Autodesk Inventor part; units mm, degrees
ref_plane "YZ Plane" through (0, 0, 0) normal (1, 0, 0) x (0, 1, 0)
ref_plane "XZ Plane" through (0, 0, 0) normal (0, 1, 0) x (-1, 0, 0)
ref_plane "XY Plane" through (0, 0, 0) normal (0, 0, 1) x (1, 0, 0)
sketch "草圖1" plane through (0, 0, 0) normal (0, 1, 0) x (-1, 0, 0)
  line L0 (21.4547, 24.4389) -> (-48.5453, 24.4389)
  line L1 (0.9998, 25.0567) -> (0.9998, 26.3567)
  line L2 (3.4998, 26.3567) -> (3.4998, 25.0567)
  line L3 (0.9998, 26.3567) -> (3.4998, 26.3567)
  line L4 (3.4998, 25.0567) -> (0.9998, 25.0567)
  line L5 (4.9998, 25.0567) -> (4.9998, 26.3567)
  line L6 (-18.5453, 30.4195) -> (12.788, 30.4195)
  line L7 (7.4998, 26.3567) -> (7.4998, 25.0567)
  line L8 (7.4998, 25.0567) -> (4.9998, 25.0567)
  line L9 (4.9998, 26.3567) -> (7.4998, 26.3567)
  line L10 (8.9998, 25.0567) -> (8.9998, 26.3567)
  line L11 (8.9998, 26.3567) -> (11.4998, 26.3567)
  line L12 (-48.5453, 23.4389) -> (-48.5453, 33.4389)
  line L13 (-38.5108, 33.4389) -> (-38.5108, 32.4389)
  line L14 (-38.5108, 32.4389) -> (-28.5108, 32.4389)
  line L15 (-28.5108, 32.4389) -> (-28.5108, 31.4389)
  line L16 (-18.5453, 31.4389) -> (-18.5453, 30.4195)
  line L17 (-28.5108, 31.4389) -> (-18.5453, 31.4389)
  line L18 (11.4998, 25.0567) -> (8.9998, 25.0567)
  line L19 (-44.5002, 26.3567) -> (-44.5002, 25.0567)
  line L20 (-44.5002, 25.0567) -> (-47.0002, 25.0567)
  line L21 (11.4998, 26.3567) -> (11.4998, 25.0567)
  line L22 (-40.5002, 26.3567) -> (-40.5002, 25.0567)
  line L23 (-40.5002, 25.0567) -> (-43.0002, 25.0567)
  line L24 (-47.0002, 25.0567) -> (-47.0002, 26.3567)
  line L25 (-47.0002, 26.3567) -> (-44.5002, 26.3567)
  line L26 (-43.0002, 26.3567) -> (-40.5002, 26.3567)
  line L27 (-36.5002, 26.3567) -> (-36.5002, 25.0567)
  line L28 (-39.0002, 26.3567) -> (-36.5002, 26.3567)
  line L29 (-39.0002, 25.0567) -> (-39.0002, 26.3567)
  line L30 (-36.5002, 25.0567) -> (-39.0002, 25.0567)
  line L31 (-43.0002, 25.0567) -> (-43.0002, 26.3567)
  line L32 (-32.5002, 26.3567) -> (-32.5002, 25.0567)
  line L33 (-32.5002, 25.0567) -> (-35.0002, 25.0567)
  line L34 (-35.0002, 26.3567) -> (-32.5002, 26.3567)
  line L35 (-35.0002, 25.0567) -> (-35.0002, 26.3567)
  line L36 (-28.5002, 26.3567) -> (-28.5002, 25.0567)
  line L37 (-28.5002, 25.0567) -> (-31.0002, 25.0567)
  line L38 (-31.0002, 26.3567) -> (-28.5002, 26.3567)
  line L39 (-31.0002, 25.0567) -> (-31.0002, 26.3567)
  line L40 (-24.5002, 26.3567) -> (-24.5002, 25.0567)
  line L41 (-24.5002, 25.0567) -> (-27.0002, 25.0567)
  line L42 (-27.0002, 25.0567) -> (-27.0002, 26.3567)
  line L43 (-27.0002, 26.3567) -> (-24.5002, 26.3567)
  line L44 (-20.5002, 26.3567) -> (-20.5002, 25.0567)
  line L45 (-20.5002, 25.0567) -> (-23.0002, 25.0567)
  line L46 (-23.0002, 26.3567) -> (-20.5002, 26.3567)
  line L47 (-23.0002, 25.0567) -> (-23.0002, 26.3567)
  line L48 (-16.5002, 26.3567) -> (-16.5002, 25.0567)
  line L49 (-19.0002, 26.3567) -> (-16.5002, 26.3567)
  line L50 (-19.0002, 25.0567) -> (-19.0002, 26.3567)
  line L51 (-16.5002, 25.0567) -> (-19.0002, 25.0567)
  line L52 (-12.5002, 26.3567) -> (-12.5002, 25.0567)
  line L53 (-15.0002, 26.3567) -> (-12.5002, 26.3567)
  line L54 (-15.0002, 25.0567) -> (-15.0002, 26.3567)
  line L55 (-12.5002, 25.0567) -> (-15.0002, 25.0567)
  line L56 (-8.5002, 26.3567) -> (-8.5002, 25.0567)
  line L57 (-8.5002, 25.0567) -> (-11.0002, 25.0567)
  line L58 (-11.0002, 25.0567) -> (-11.0002, 26.3567)
  line L59 (-11.0002, 26.3567) -> (-8.5002, 26.3567)
  line L60 (-4.5002, 25.0567) -> (-7.0002, 25.0567)
  line L61 (-7.0002, 26.3567) -> (-4.5002, 26.3567)
  line L62 (-7.0002, 25.0567) -> (-7.0002, 26.3567)
  line L63 (-4.5002, 26.3567) -> (-4.5002, 25.0567)
  line L64 (-3.0002, 25.0567) -> (-3.0002, 26.3567)
  line L65 (-0.5002, 25.0567) -> (-3.0002, 25.0567)
  line L66 (-3.0002, 26.3567) -> (-0.5002, 26.3567)
  line L67 (-0.5002, 26.3567) -> (-0.5002, 25.0567)
  line L68 (-48.5453, 33.4389) -> (-38.5108, 33.4389)
  line L69 (21.4547, 24.4389) -> (12.788, 30.4195)
  line L70 (12.2792, 28.0771) -> (12.2792, 25.0771)
  line L71 (14.7792, 28.0771) -> (12.2792, 28.0771)
  line L72 (12.2792, 25.0771) -> (14.7792, 25.0771)
  line L73 (14.7792, 25.0771) -> (14.7792, 28.0771)
  line L74 (-48.5453, 33.4389) -> (-48.5453, 23.4389)
  line L75 (-48.5453, 23.4389) -> (-48.5453, 24.4389)
  line L76 (-48.5453, 24.4389) -> (21.4547, 24.4389)
  line L77 (21.4547, 24.4389) -> (21.4547, 23.4389)
  line L78 (21.4547, 23.4389) -> (-48.5453, 23.4389)
  point P0 (34.4342, -20.4461)
  dimension "d19" = 2.5
  dimension "d20" = 3
  dimension "d26" = 70
  dimension "d27" = 10
extrude "擠出1" add sketch "草圖1" along normal blind 2
properties part number "援助旁邊4跟"
Design review of the part built by this model. Coordinates are the model's own, in mm. A direction names the side the tool comes from. Coordinates: 2 decimals unless noted, no trailing zeros. Order: outer loops, then holes, each group sorted by start corner. A loop starts at its lowest first (then second) coordinate and runs counter-clockwise, first axis right, second up. Notation, with made-up numbers: M -32.5,70.25 L 19.5,70.25 A18 ccw 19.5,75.25 Z; hole C 61.5,82 d3. An arc over 180 degrees is marked long. Use a Markdown table: item, result.
(1) Add section A-A (x = 34). Give the boundary of the cut face in (y, z), then the cut area to 3 significant figures.
Worked answers:
| item | result |
|---|---|
| outline | M 0,23.44 L 2,23.44 L 2,25.06 L 0,25.06 Z; M 0,26.36 L 2,26.36 L 2,32.44 L 0,32.44 Z |
| area | 15.4 mm2 |
(2) Draft analysis for pull direction Z (two halves, no side actions). For faces 1 (the flat face through (22, 1, 26.357)), 2 (the flat face through (-17.18, 0.99, 27.39)), state which applies: released by +Z, released by -Z, zero draft, split by the parting line, or undercut.
Worked answers:
| item | result |
|---|---|
| face 1 | undercut |
| face 2 | released by +Z |
(3) Add section B-B (z = 27). Give the boundary of the cut face in (x, y).
Worked answers:
| item | result |
|---|---|
| outline | M -17.74,0 L -14.78,0 L -14.78,2 L -17.74,2 Z; M -12.28,0 L 48.55,0 L 48.55,2 L -12.28,2 Z |
(4) For faces 3 (the flat face through (34, 1, 32.439)), 4 (the flat face through (15, 1, 26)), list the 3-axis set-ups (+Z, -Z, +X, -X, +Y, -Y) from which the entire face can be reached by the end or side of a thin tool; tool diameter is ignored.
Worked answers:
| item | result |
|---|---|
| face 3 | +Z, -X, +Y, -Y |
| face 4 | +Y, -Y |
(5) Add section D-D (z = 29.5). Give the boundary of the cut face in (x, y), then the cut area to 3 significant figures.
Worked answers:
| item | result |
|---|---|
| outline | M -14.12,0 L 48.55,0 L 48.55,2 L -14.12,2 Z |
| area | 125 mm2 |
(6) Add section C-C (y = 1.05). Count the separate pieces of the cut face and the enclosed holes in it, then the cut area to 3 significant figures.
Worked answers:
| item | result |
|---|---|
| separate pieces | 1 |
| enclosed holes | 16 |
| area | 467 mm2 |
(7) Wall thickness on probe 1 along Z at (x, y) = (-2.5, 0.9); probe 2 along Z at (x, y) = (26, 1.45); probe 3 along Z at (x, y) = (-8, 0.65): over which ranges is each line inside the solid? List them lowest first.
Worked answers:
| item | result |
|---|---|
| probe 1 | z = 23.44 to 25.06, 26.36 to 30.42 |
| probe 2 | z = 23.44 to 25.06, 26.36 to 31.44 |
| probe 3 | z = 23.44 to 30.42 |
(8) For P1, Ø0.7, axis at y = 1, z = 26, coming from the -X side; P2, Ø0.6, axis at x = 24, y = 1.5, coming from the +Z side; P3, Ø0.6, axis at x = -13.5, y = 1, coming from the +Z side, all flat-tipped, find the tip position at first contact; note any pin that passes through.
Worked answers:
| item | result |
|---|---|
| P1 | stops at x = -19.7 |
| P2 | stops at z = 31.44 |
| P3 | stops at z = 30.14 |
